Work out the finished part from the listing and answer in its coordinate system (mm). A direction names the side the tool comes from. Coordinates: 2 decimals unless noted, no trailing zeros. Order: outer loops, then holes, each group sorted by start corner. A loop starts at its lowest first (then second) coordinate and runs counter-clockwise, first axis right, second up. Notation, with made-up numbers: (-37, 38.25) - (-25, 38.25) arc R22 cw to (-25, 57.25) - close; hole circle Ø6 at (-17, 3). An arc over 180 degrees is marked (long way). Use CSV: the item, a comma, the result in double quotes. Start each with the question number.
from build123d import *

# Parameters (mm, degrees)
F0_W      = 107.4284315109
F0_H      = 51.8054459244
F1_DEPTH  = 6.35
F2_W      = 2.7584051713
F2_H      = 16.6592616588
F3_DEPTH  = 54.102
F4_R      = 4.9057005628
F5_DEPTH  = 45.4490629414
F6_R      = 38.9203036593
F7_DEPTH  = 6.35
F8_DEPTH  = 16.51
F9_R      = 3.1625742778
F10_DEPTH = 45.4490629414


with BuildPart() as f1:
    # F0 (on Top) → F1 (new body)
    with BuildSketch(Plane.XY):
        with Locations((1.9887797534, 4.2384741828)):
            Rectangle(F0_W, F0_H)
    extrude(amount=F1_DEPTH)

    # F2 (on face) → F3 (join)
    with BuildSketch(Plane.XY.offset(6.35)):
        with Locations((-7.6565756463, 8.3296308294)):
            Rectangle(F2_W, F2_H)
    extrude(amount=F3_DEPTH)

    # F4 (on face) → F5 (cut, through all)
    with BuildSketch(Plane.YZ.offset(-6.2773730606)):
        with Locations((8.3296308294, 50.6100766361)):
            Circle(F4_R)
    extrude(amount=-F5_DEPTH, mode=Mode.SUBTRACT)

    # F6 (on face) → F7 (join)
    with BuildSketch(Plane(origin=(-9.0357782319, 0, 0), x_dir=(0, -1, 0), z_dir=(-1, 0, 0))):
        with Locations((-8.3296308294, 81.4679414034)):
            Circle(F6_R)
    extrude(amount=F7_DEPTH)

    # F8 (add): a face of the model
    f8_faces = [f1.faces().sort_by_distance(p)[0] for p in [
        (-9.0357782319, 8.3296308294, 50.6100766361),
    ]]
    extrude(f8_faces, amount=F8_DEPTH)

    # F9 (on face) → F10 (cut, through all)
    with BuildSketch(Plane.YZ.offset(-6.2773730606)):
        with Locations((6.9233309478, 16.4294000715)):
            Circle(F9_R)
    extrude(amount=-F10_DEPTH, mode=Mode.SUBTRACT)


solid = f1.part
1) Straight lines are drawn through the part: line 1 (X direction, y = -9, z = 49); line 2 (Z direction, x = -42, y = -0.5); line 3 (X direction, y = 7.5, z = 42.5). For each, find the intervals that lie inside material, in ascending order. Write a range as [from, to].
2) The part is cut by section D-D on x = 48. Determine the outline of the cut face in (y, z).
3) The part is cut by section C-C on z = 24. Determine the outline of the cut face in (x, y), plus the area to 3 significant figures.
4) The part is cut by section A-A on y = -2. Determine the outline of the cut face in (x, z).
5) For faces 4 (the face through (7.474, 8, 51)), 5 (the face through (-8, 0, 33)), 6 (the face through (-15.386, 9, 82)), determine the directions among +Z, -Z, +X, -X, +Y, -Y from which every point of the face is accessible in a straight line to the end or side of a thin tool.
6) The part is cut by section B-B on y = -17. Determine the outline of the cut face in (x, z).
7) Flat-ended cylindrical pins translate along their axes: P1, Ø8, axis at x = -33, y = 34.5, coming from the +Z side; P2, Ø23, axis at y = 19.5, z = 99.5, coming from the +X side; P3, Ø5, axis at x = -10, y = 21, coming from the -Z side; P4, Ø8, axis at x = 29, y = 4, coming from the +Z side. Find the tip coordinate at first contact, or state that the pin passes through.
8) For a pull along Z with two mould halves and no side action, classify faces 1 (the face through (-8, 16.659, 33)), 2 (the face through (-8, 8, 60.452)), 3 (the face through (0.502, 7.691, 55.474)) as +Z half, -Z half, draft (parallel to the pull), parting line (faces both ways), or undercut.
Answer key:
1,line 1,"[-15.39, -9.04]"
1,line 2,"[0, 6.35]"
1,line 3,"[-9.04, -6.28]"
2,outline,"(-21.66, 0) - (30.14, 0) - (30.14, 6.35) - (-21.66, 6.35) - close"
3,outline,"(-9.04, 0) - (-6.28, 0) - (-6.28, 16.66) - (-9.04, 16.66) - close"
3,area,"46.0 mm^2"
4,outline,"(-51.73, 0) - (55.7, 0) - (55.7, 6.35) - (-51.73, 6.35) - close; (-15.39, 43.94) - (-9.04, 43.94) - (-9.04, 118.99) - (-15.39, 118.99) - close"
5,face 4,"+Z, +X, +Y, -Y"
5,face 5,"+Z, +X, -Y"
5,face 6,"+Z, -X, +Y, -Y"
6,outline,"(-51.73, 0) - (55.7, 0) - (55.7, 6.35) - (-51.73, 6.35) - close; (-15.39, 51.92) - (-9.04, 51.92) - (-9.04, 111.02) - (-15.39, 111.02) - close"
7,P1,"through"
7,P2,"x = -9.04"
7,P3,"z = 0"
7,P4,"z = 6.35"
8,face 1,"draft"
8,face 2,"+Z half"
8,face 3,"undercut"
